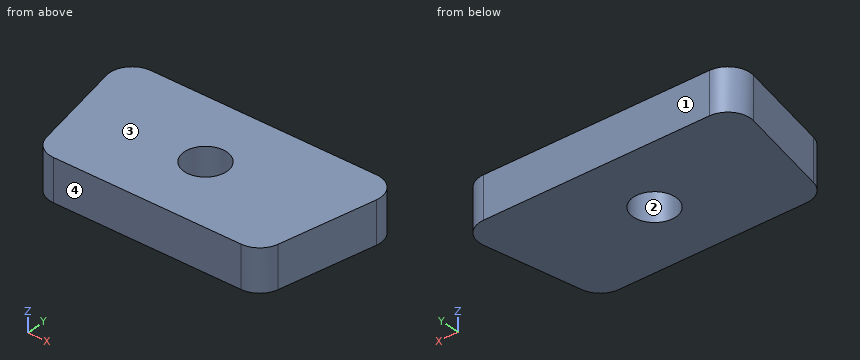
```python
from build123d import *

# Parameters (mm, degrees)
F2_DEPTH = 9.525
F1_R     = 4.826
F3_DEPTH = 9.525
F4_R     = 5.08


with BuildPart() as f2:
    # F0 (on Top) → F2 (new body)
    with BuildSketch(Plane.XY):
        Polygon((31.75, 31.75), (0, 31.75), (-31.75, 31.75), (-25.4, 0), (0, 0), (25.4, 0), align=None)
    extrude(amount=F2_DEPTH)

    # F1 (on face) → F3 (cut, through all)
    with BuildSketch(Plane.XY):
        with Locations((0, 15.875)):
            Circle(F1_R)
    extrude(amount=F3_DEPTH, mode=Mode.SUBTRACT)

    # F4
    f4_edges = [f2.edges().sort_by_distance(p)[0] for p in [
        (-31.75, 31.75, 4.7625),
        (31.75, 31.75, 4.7625),
        (25.4, 0, 4.7625),
        (-25.4, 0, 4.7625),
    ]]
    fillet(f4_edges, radius=F4_R)


solid = f2.part
```
The model under review builds one solid part; all positions refer to its coordinate system, in mm. Face numbers are marked on the shaded views. Give positions to 0.01 mm unless a question says otherwise; leave off trailing zeros. Write each loop counter-clockwise with the first axis right and the second up, starting at its lowest first coordinate (ties: lowest second). Pieces come first, ordered by that corner, then holes.
(1) The part is to be moulded in two halves that separate along Y. For the marked faces 1, 2, 3 and 4, say which applies: released by +Y, released by -Y, zero draft, split by the parting line, or undercut.
(2) Consider section A-A, the plane x = 0. Give the boundary of the cut face in (y, z) (3 decimals).
(3) To check wall thickness, follow L1, parallel to Y at x = 0, z = 2.75; L2, parallel to Y at x = 3, z = 1.5; L3, parallel to X at y = 12.5, z = 8.5. State the ranges of each line that lie inside material, in increasing order.
(4) For P1, Ø1.5, axis at y = 28, z = 1, coming from the -X side; P2, Ø7.5, axis at x = 0, y = 15.875, coming from the +Z side, all flat-tipped, find the tip position at first contact; note any pin that passes through.
(5) Consider section D-D, the plane y = 23.5. Give the boundary of the cut face in (x, z) (3 decimals).
(6) Consider section C-C, the plane z = 3.25. Give the boundary of the cut face in (x, y) (3 decimals).
(7) Consider section B-B, the plane y = 19. Give the boundary of the cut face in (x, z) (3 decimals).
Returned:
1. face 1: released by +Y
1. face 2: undercut
1. face 3: zero draft
1. face 4: released by -Y
2. outline: (0, 0) - (11.049, 0) - (11.049, 9.525) - (0, 9.525) - close; (20.701, 0) - (31.75, 0) - (31.75, 9.525) - (20.701, 9.525) - close
3. L1: y = 0 to 11.05, 20.7 to 31.75
3. L2: y = 0 to 12.09, 19.66 to 31.75
3. L3: x = -27.9 to -3.45, 3.45 to 27.9
4. P1: stops at x = -30.6
4. P2: passes through
5. outline: (-30.1, 0) - (30.1, 0) - (30.1, 9.525) - (-30.1, 9.525) - close
6. outline: (-30.535, 25.674) - (-26.217, 4.084) arc R5.08 ccw to (-21.235, 0) - (21.235, 0) arc R5.08 ccw to (26.217, 4.084) - (30.535, 25.674) arc R5.08 ccw to (25.553, 31.75) - (-25.553, 31.75) arc R5.08 ccw to start; hole circle Ø9.652 at (0, 15.875)
7. outline: (-29.2, 0) - (-3.678, 0) - (-3.678, 9.525) - (-29.2, 9.525) - close; (3.678, 0) - (29.2, 0) - (29.2, 9.525) - (3.678, 9.525) - close
